from build123d import *

# Parameters (mm, degrees)
SKETCH1_W           = 9.8
SKETCH1_H           = 4.7
SKETCH1_H_2         = 0.1
SKETCH1_W_2         = 0.1
SKETCH1_H_3         = 10.9
SKETCH1_W_3         = 0.2
BOSS_EXTRUDE1_DEPTH = 0.3


with BuildPart() as part:
    # Sketch1 → Boss-Extrude1 (new body)
    with BuildSketch(Plane(origin=(0, 0, 0), x_dir=(1, 0, 0), z_dir=(0, 1, 0))):
        with Locations((-5.25, 13.35)):
            Rectangle(SKETCH1_W, SKETCH1_H)
        with Locations((5.25, 13.35)):
            Rectangle(SKETCH1_W, SKETCH1_H)
        with Locations((-5.25, 10.95)):
            Rectangle(SKETCH1_W, SKETCH1_H_2)
        with Locations((5.25, 10.95)):
            Rectangle(SKETCH1_W, SKETCH1_H_2)
        Polygon((-0.35, 11), (-0.35, 10.9), (0.35, 10.9), (0.35, 11), (0.25, 11), (-0.25, 11), align=None)
        Polygon((-10.15, 10.9), (-10.15, 0), (10.15, 0), (10.15, 10.9), (0.35, 10.9), (-0.35, 10.9), align=None)
        with Locations((-10.2, 5.45)):
            Rectangle(SKETCH1_W_2, SKETCH1_H_3)
        with Locations((-10.35, 5.45)):
            Rectangle(SKETCH1_W_3, SKETCH1_H_3)
        with Locations((10.35, 5.45)):
            Rectangle(SKETCH1_W_3, SKETCH1_H_3)
        with Locations((10.2, 5.45)):
            Rectangle(SKETCH1_W_2, SKETCH1_H_3)
    extrude(amount=BOSS_EXTRUDE1_DEPTH)


solid = part.part
The model under review builds one solid part; all positions refer to its coordinate system, in mm. Coordinates: 2 decimals unless noted, no trailing zeros. Loops run counter-clockwise (first coordinate to the right, second up) from the corner with the lowest first, then second, coordinate; pieces in that order, holes last. Notation, with made-up numbers: (78.5, -21) -> (82.5, -21) arc R24 ccw to (82.5, 5) -> close; hole circle Ø5 at (50.5, -17.75). An arc over 180 degrees is marked (long way). Use a Markdown table: item, result. Add a question column.
1. To check wall thickness, follow line 1 (X direction, y = 0.15, z = -14.5). State the ranges of the line that lie inside material, in increasing order.
2. Add section A-A on z = -13.75. Write out the cut boundary in (x, y).
3. Add section B-B on y = 0.25. Write out the cut boundary in (x, z), plus the area to 3 significant figures.
Returned:
| question | item | result |
|---|---|---|
| 1 | line 1 | x = -10.15 to -0.35, 0.35 to 10.15 |
| 2 | outline | (-10.15, 0) -> (-0.35, 0) -> (-0.35, 0.3) -> (-10.15, 0.3) -> close; (0.35, 0) -> (10.15, 0) -> (10.15, 0.3) -> (0.35, 0.3) -> close |
| 3 | outline | (-10.45, -10.9) -> (-10.15, -10.9) -> (-10.15, -15.7) -> (-0.35, -15.7) -> (-0.35, -11) -> (0.35, -11) -> (0.35, -15.7) -> (10.15, -15.7) -> (10.15, -10.9) -> (10.45, -10.9) -> (10.45, 0) -> (-10.45, 0) -> close |
| 3 | area | 322 mm² |
